from build123d import *

# Parameters (mm, degrees)
F1_DEPTH       = 10
F3_D           = 4.4
F3_CBORE_D     = 8.25
F3_CBORE_DEPTH = 4
F5_D           = 4.4


# Not quite as in the source:
# - a feature names something its author has since deleted; it is built from what else it names


with BuildPart() as f1:
    # F0 (on Front) → F1 (new body)
    with BuildSketch(Plane.XZ):
        Polygon((-80, 10), (0, 10), (0, 20), (-70, 20), align=None)
        Polygon((-70, 0), (0, 0), (0, 10), (-80, 10), align=None)
    extrude(amount=F1_DEPTH)

    # F3 (through all)
    with Locations(Plane.XZ.offset(10)):
        with Locations((-20, 5), (-60, 5)):
            CounterBoreHole(F3_D / 2, F3_CBORE_D / 2, F3_CBORE_DEPTH)

    # F5 (through all)
    with Locations(Plane.XZ.offset(10)):
        with Locations((-60, 15), (-20, 15)):
            Hole(F5_D / 2)


solid = f1.part
Geometry check sheet. Reference: the model listing, model coordinates, mm. A direction names the side the tool comes from. Give positions to 0.01 mm unless a question says otherwise; leave off trailing zeros. Loops run counter-clockwise (first coordinate to the right, second up) from the corner with the lowest first, then second, coordinate; pieces in that order, holes last.
(1) Section check D-D on y = -2. Record the cut outline in (x, z), then the cut area to 3 significant figures.
From the geometry:
outline: (-80, 10) - (-70, 0) - (0, 0) - (0, 20) - (-70, 20) - close; hole circle Ø4.4 at (-60, 5); hole circle Ø4.4 at (-60, 15); hole circle Ø4.4 at (-20, 5); hole circle Ø4.4 at (-20, 15)
area: 1,440 mm2
(2) Set-up check for faces 4 (the cylindrical face through (-62.1, -2.96, 5.66)), 5 (the cylindrical face through (-61, -8, 1)): record each of +Z, -Z, +X, -X, +Y, -Y from which the full face is reachable in a straight line by a thin tool's end or side.
From the geometry:
face 4: +Y, -Y
face 5: -Y
(3) Depth check by flat-ended pin: pin 1 Ø2.5 at (x, z) = (-20, 15) entering from +Y; pin 2 Ø5 at (x, z) = (-20, 5) entering from -Y; pin 3 Ø1 at (y, z) = (-8.5, 4) entering from -X. Enter the tip coordinate at first touch or a pass-through.
From the geometry:
pin 1: passes through
pin 2: stops at y = -6
pin 3: stops at x = -74.5
(4) Thickness scan on L1, parallel to Z at x = -20, y = -7.4 (3 decimals); L2, parallel to Z at x = -60, y = -1.45; L3, parallel to X at y = -3, z = 4. Record the ranges inside material, lowest first.
From the geometry:
L1: z = 0 to 0.875, 9.125 to 12.8, 17.2 to 20
L2: z = 0 to 2.8, 7.2 to 12.8, 17.2 to 20
L3: x = -74 to -61.96, -58.04 to -21.96, -18.04 to 0
(5) Section check C-C on x = -60. Record the cut outline in (y, z) (3 decimals).
From the geometry:
outline: (-10, 0) - (0, 0) - (0, 2.8) - (-6, 2.8) - (-6, 0.875) - (-10, 0.875) - close; (-10, 9.125) - (-6, 9.125) - (-6, 7.2) - (0, 7.2) - (0, 12.8) - (-10, 12.8) - close; (-10, 17.2) - (0, 17.2) - (0, 20) - (-10, 20) - close
(6) Release check for a two-part mould opening along Z. For faces 1 (the cylindrical face through (-62.032, -4.93, 14.157)), 2 (the flat face through (-75, -5, 5)), 3 (the flat face through (-35, -5, 20)) record: released by +Z, released by -Z, zero draft, split by the parting line, or undercut.
From the geometry:
face 1: undercut
face 2: released by -Z
face 3: released by +Z
(7) Section check A-A on y = -8.75. Record the cut outline in (x, z) (3 decimals).
From the geometry:
outline: (-80, 10) - (-70, 0) - (0, 0) - (0, 20) - (-70, 20) - close; hole circle Ø8.25 at (-60, 5); hole circle Ø4.4 at (-60, 15); hole circle Ø8.25 at (-20, 5); hole circle Ø4.4 at (-20, 15)
(8) Section check B-B on z = 5. Record the cut outline in (x, y) (3 decimals), then the cut area to 3 significant figures.
From the geometry:
outline: (-75, -10) - (-64.125, -10) - (-64.125, -6) - (-62.2, -6) - (-62.2, 0) - (-75, 0) - close; (-57.8, -6) - (-55.875, -6) - (-55.875, -10) - (-24.125, -10) - (-24.125, -6) - (-22.2, -6) - (-22.2, 0) - (-57.8, 0) - close; (-17.8, -6) - (-15.875, -6) - (-15.875, -10) - (0, -10) - (0, 0) - (-17.8, 0) - close
area: 631 mm2
